from build123d import *

# Parameters (mm, degrees)
F0_R     = 10.95
F1_DEPTH = 2.4
F2_R     = 4.225
F3_DEPTH = 4.2
F4_R     = 1
F5_R     = 6
F6_DEPTH = 1
F7_R     = 1
F8_SIZE  = 0.4


with BuildPart() as f1:
    # F0 (on Top) → F1 (new body)
    with BuildSketch(Plane.XY):
        Circle(F0_R)
    extrude(amount=F1_DEPTH)

    # F2 (on face) → F3 (join)
    with BuildSketch(Plane.XY.offset(2.4)):
        Circle(F2_R)
    extrude(amount=F3_DEPTH)

    # F4
    f4_edges = [f1.edges().sort_by_distance(p)[0] for p in [
        (-10.95, 0, 2.4),
    ]]
    fillet(f4_edges, radius=F4_R)

    # F5 (on face) → F6 (join)
    with BuildSketch(Plane.XY.offset(2.4)):
        Circle(F5_R)
    extrude(amount=F6_DEPTH)

    # F7
    f7_edges = [f1.edges().sort_by_distance(p)[0] for p in [
        (-10.95, 0, 0),
    ]]
    fillet(f7_edges, radius=F7_R)

    # F8
    f8_edges = [f1.edges().sort_by_distance(p)[0] for p in [
        (-4.225, 0, 6.6),
    ]]
    chamfer(f8_edges, length=F8_SIZE)


solid = f1.part
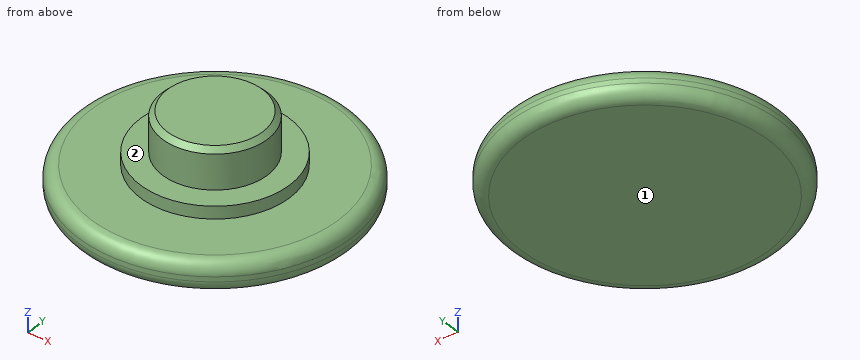
For this review, take the finished solid that the model builds, in its own axes (mm). Face numbers are marked on the shaded views. A direction names the side the tool comes from. Coordinates: 2 decimals unless noted, no trailing zeros. Write each loop counter-clockwise with the first axis right and the second up, starting at its lowest first coordinate (ties: lowest second). Pieces come first, ordered by that corner, then holes. Notation, with made-up numbers: (64, -30) -> (115, -30) arc R27 ccw to (115, 0) -> close; hole circle Ø1 at (-3, 32.25). An arc over 180 degrees is marked (long way). Write each question's results on one line, items separated by ' | '. Start each with the question number.
1) For the marked faces 1 and 2, list the 3-axis set-ups (+Z, -Z, +X, -X, +Y, -Y) from which the entire face can be reached by the end or side of a thin tool; tool diameter is ignored.
2) Insertion check: pin 1 (3 mm diameter, centred on y = -7, z = 2.5, fed in from +X). The pin has a flat end and moves straight along its axis. Give the tip position at first contact, or say it passes through.
3) Consider section C-C (z = 5.75). Write out the cut boundary in (x, y) (3 decimals).
4) Consider section A-A (x = 0). Write out the cut boundary in (y, z) (3 decimals), plus the area to 3 significant figures.
5) Wall thickness on L1, parallel to Z at x = -5.25, y = 7; L2, parallel to Y at x = 0.25, z = 2.5; L3, parallel to Y at x = 0.25, z = 6: over which ranges is each line inside the solid? List them lowest first. Write a range as [from, to].
6) Consider section D-D (z = 2). Write out the cut boundary in (x, y).
Geometry says:
1) face 1: -Z, +X, -X, +Y, -Y | face 2: +Z
2) pin 1: x = 9.28
3) outline: circle Ø8.45 at (0, 0)
4) outline: (-10.95, 1) arc R1 ccw to (-9.95, 0) -> (9.95, 0) arc R1 ccw to (10.95, 1) -> (10.95, 1.4) arc R1 ccw to (9.95, 2.4) -> (6, 2.4) -> (6, 3.4) -> (4.225, 3.4) -> (4.225, 6.2) -> (3.825, 6.6) -> (-3.825, 6.6) -> (-4.225, 6.2) -> (-4.225, 3.4) -> (-6, 3.4) -> (-6, 2.4) -> (-9.95, 2.4) arc R1 ccw to (-10.95, 1.4) -> close | area: 90.6 mm^2
5) L1: [0, 2.4] | L2: [-5.99, 5.99] | L3: [-4.22, 4.22]
6) outline: circle Ø21.5 at (0, 0)
